The listing builds one solid part. Answer for the finished solid, in the listing's coordinates (mm). Face numbers are marked on the shaded views. A direction names the side the tool comes from. Give positions to 0.01 mm unless a question says otherwise; leave off trailing zeros. Write each loop counter-clockwise with the first axis right and the second up, starting at its lowest first coordinate (ties: lowest second). Pieces come first, ordered by that corner, then holes. Notation, with made-up numbers: M -25,-17 L 26,-17 A16 ccw 26,-1 Z; hole C 78,79 d2. An arc over 180 degrees is marked long. Return JSON: item names as keys, results as strings.
from build123d import *

# Parameters (mm, degrees)
F1_DEPTH     = 25.4
F2_R         = 9.525
F3_DEPTH     = 42.7816898715
F4_R         = 25.39999
F5_R         = 3.175
F6_W         = 5.0767767243
F6_H         = 5.0767767243
F7_DEPTH     = 3.175
F8_T1_DEPTH  = 142.613798458
F8_T3_DEPTH  = 25.40001
F8_T5_DEPTH  = 44.45
F8_T7_DEPTH  = 25.40001
F8_T9_DEPTH  = 2e-05
F8_T12_ANGLE = 90
F8_T14_ANGLE = 55
F8_T16_ANGLE = 55
F8_T18_ANGLE = 90
F8_T20_ANGLE = 90
F8_T22_ANGLE = 90
F8_T24_ANGLE = 55
F8_T26_ANGLE = 90
F8_T28_ANGLE = 90
F8_T30_ANGLE = 90
F8_T32_ANGLE = 55
F8_T34_ANGLE = 90


# Not quite as in the source:
# - a fillet or chamfer that OpenCascade refuses, or shapes differently, is made with other operations: its cross-section is extruded or revolved along the edge and cut away or added
# - a fillet or chamfer is up to 0.001 mm smaller than in the source, because OpenCascade refuses the exact size


with BuildPart() as f1:
    # F0 (on Front) → F1 (new body, symmetric)
    with BuildSketch(Plane.XZ):
        with BuildLine():
            Line((118.9895820573, 10.6313137069), (-26.7992164007, 10.6313137069))
            Line((-26.7992164007, 10.6313137069), (-26.7992164007, -2.0686862931))
            Line((-26.7992164007, -2.0686862931), (118.9895820573, -2.0686862931))
            ThreePointArc((118.9895820573, -2.0686862931), (130.7179968335, 0.8012385441), (139.7960439822, 8.7624722235))
            Line((139.7960439822, 8.7624722235), (168.9337269489, 50.3753960734))
            Line((168.9337269489, 50.3753960734), (158.5304959864, 57.6598168151))
            Line((158.5304959864, 57.6598168151), (129.3928130198, 16.0468929652))
            ThreePointArc((129.3928130198, 16.0468929652), (124.8537894454, 12.0662761255), (118.9895820573, 10.6313137069))
        make_face()
    extrude(amount=F1_DEPTH, both=True)

    # F2 (on face) → F3 (cut, through all)
    with BuildSketch(Plane(origin=(79.2843072841, 0, -55.515469622), x_dir=(0, -1, 0), z_dir=(-0.8191520443, 0, 0.5735764364))):
        with Locations((0, 115.9365137582)):
            Circle(F2_R)
    extrude(amount=-F3_DEPTH, mode=Mode.SUBTRACT)

    # F4 (radius 25.4 in the source; OpenCascade refuses exactly that, so slightly less here)
    f4_edges = [f1.edges().sort_by_distance(p)[0] for p in [
        (163.732111, 25.4, 54.017606),
        (163.732111, -25.4, 54.017606),
    ]]
    fillet(f4_edges, radius=F4_R)

    # F5
    f5_edges = [f1.edges().sort_by_distance(p)[0] for p in [
        (-26.799216, -25.4, 4.281314),
        (-26.799216, 25.4, 4.281314),
    ]]
    fillet(f5_edges, radius=F5_R)

    # F6 (on face) → F7 (cut)
    with BuildSketch(Plane(origin=(0, 0, -2.0686862931), x_dir=(1, 0, 0), z_dir=(0, 0, -1))):
        with Locations((4.9507835993, 0)):
            Rectangle(F6_W, F6_H)
    extrude(amount=-F7_DEPTH, mode=Mode.SUBTRACT)

    # F8: fillet of radius 3.175 on 24 edges, made by hand

    # F8_s2 → F8_t1 (cut)
    with BuildSketch(Plane.YZ.offset(-23.6242164007)):
        with BuildLine():
            ThreePointArc((25.4, 7.4563137069), (24.4700640303, 9.7013777371), (22.225, 10.6313137069))
            Line((22.225, 10.6313137069), (25.4, 10.6313137069))
            Line((25.4, 10.6313137069), (25.4, 7.4563137069))
        make_face()
        with BuildLine():
            ThreePointArc((-22.225, 10.6313137069), (-24.4700640303, 9.7013777371), (-25.4, 7.4563137069))
            Line((-25.4, 7.4563137069), (-25.4, 10.6313137069))
            Line((-25.4, 10.6313137069), (-22.225, 10.6313137069))
        make_face()
        with BuildLine():
            ThreePointArc((-22.225, -2.0686862931), (-24.4700640303, -1.1387503234), (-25.4, 1.1063137069))
            Line((-25.4, 1.1063137069), (-25.4, -2.0686862931))
            Line((-25.4, -2.0686862931), (-22.225, -2.0686862931))
        make_face()
        with BuildLine():
            ThreePointArc((25.4, 1.1063137069), (24.4700640303, -1.1387503234), (22.225, -2.0686862931))
            Line((22.225, -2.0686862931), (25.4, -2.0686862931))
            Line((25.4, -2.0686862931), (25.4, 1.1063137069))
        make_face()
    extrude(amount=F8_T1_DEPTH, mode=Mode.SUBTRACT)

    # F8_s4 → F8_t3 (cut)
    with BuildSketch(Plane(origin=(64.6773529548, 0, 92.3688327037), x_dir=(0, 1, 0), z_dir=(-0.5735764364, 0, -0.8191520443))):
        with BuildLine():
            ThreePointArc((25.4, 99.96326762), (24.4700640303, 97.7182035897), (22.225, 96.78826762))
            Line((22.225, 96.78826762), (25.4, 96.78826762))
            Line((25.4, 96.78826762), (25.4, 99.96326762))
        make_face()
        with BuildLine():
            ThreePointArc((-22.225, 96.78826762), (-24.4700640303, 97.7182035897), (-25.4, 99.96326762))
            Line((-25.4, 99.96326762), (-25.4, 96.78826762))
            Line((-25.4, 96.78826762), (-22.225, 96.78826762))
        make_face()
    extrude(amount=F8_T3_DEPTH, mode=Mode.SUBTRACT)

    # F8_s6 → F8_t5 (cut)
    with BuildSketch(Plane.XZ.offset(-22.225)):
        with BuildLine():
            ThreePointArc((-23.6242164007, 10.6313137069), (-25.869280431, 9.7013777371), (-26.7992164007, 7.4563137069))
            Line((-26.7992164007, 7.4563137069), (-26.7992164007, 10.6313137069))
            Line((-26.7992164007, 10.6313137069), (-23.6242164007, 10.6313137069))
        make_face()
        with BuildLine():
            ThreePointArc((-23.6242164007, -2.0686862931), (-25.869280431, -1.1387503234), (-26.7992164007, 1.1063137069))
            Line((-26.7992164007, 1.1063137069), (-26.7992164007, -2.0686862931))
            Line((-26.7992164007, -2.0686862931), (-23.6242164007, -2.0686862931))
        make_face()
    extrude(amount=F8_T5_DEPTH, mode=Mode.SUBTRACT)

    # F8_s8 → F8_t7 (cut)
    with BuildSketch(Plane(origin=(50.1085057357, 0, 71.5623625873), x_dir=(0, 1, 0), z_dir=(0.5735764364, 0, 0.8191520443))):
        with BuildLine():
            ThreePointArc((25.4, -106.31326762), (24.4700640303, -108.5583316502), (22.225, -109.48826762))
            Line((22.225, -109.48826762), (25.4, -109.48826762))
            Line((25.4, -109.48826762), (25.4, -106.31326762))
        make_face()
        with BuildLine():
            ThreePointArc((-22.225, -109.48826762), (-24.4700640303, -108.5583316502), (-25.4, -106.31326762))
            Line((-25.4, -106.31326762), (-25.4, -109.48826762))
            Line((-25.4, -109.48826762), (-22.225, -109.48826762))
        make_face()
    extrude(amount=F8_T7_DEPTH, mode=Mode.SUBTRACT)

    # F8_s10 → F8_t9 (cut)
    with BuildSketch(Plane.XZ.offset(-1e-05)):
        with BuildLine():
            ThreePointArc((167.1126217635, 47.7745883328), (167.6385786386, 50.1470264823), (166.3329192083, 52.1965012588))
            Line((166.3329192083, 52.1965012588), (168.9337269489, 50.3753960734))
            Line((168.9337269489, 50.3753960734), (167.1126217635, 47.7745883328))
        make_face()
        with BuildLine():
            ThreePointArc((156.709390801, 55.0590090745), (158.7588655775, 56.3646685049), (161.131303727, 55.8387116297))
            Line((161.131303727, 55.8387116297), (158.5304959864, 57.6598168151))
            Line((158.5304959864, 57.6598168151), (156.709390801, 55.0590090745))
        make_face()
    extrude(amount=F8_T9_DEPTH, mode=Mode.SUBTRACT)

    # F8_s11 → F8_t12 (revolve, cut)
    with BuildSketch(Plane(origin=(64.6773529548, 0, 92.3688327037), x_dir=(0, 1, 0), z_dir=(-0.5735764364, 0, -0.8191520443))):
        with BuildLine():
            ThreePointArc((25.4, 99.96326762), (24.4700640303, 97.7182035897), (22.225, 96.78826762))
            Line((22.225, 96.78826762), (25.4, 96.78826762))
            Line((25.4, 96.78826762), (25.4, 99.96326762))
        make_face()
    revolve(axis=Axis((143.9616602388, 1e-05, 36.8533630817), (0.8191520443, 0, -0.5735764364)), revolution_arc=F8_T12_ANGLE, mode=Mode.SUBTRACT)

    # F8_s13 → F8_t14 (revolve, cut)
    with BuildSketch(Plane.YZ.offset(118.9895820573)):
        with BuildLine():
            ThreePointArc((25.4, 1.1063137069), (24.4700640303, -1.1387503234), (22.225, -2.0686862931))
            Line((22.225, -2.0686862931), (25.4, -2.0686862931))
            Line((25.4, -2.0686862931), (25.4, 1.1063137069))
        make_face()
    revolve(axis=Axis((118.9895820573, 25.4, 23.3313137069), (0, -1, 0)), revolution_arc=F8_T14_ANGLE, mode=Mode.SUBTRACT)

    # F8_s15 → F8_t16 (revolve, cut)
    with BuildSketch(Plane(origin=(50.1085057357, 0, 71.5623625873), x_dir=(0, 1, 0), z_dir=(0.5735764364, 0, 0.8191520443))):
        with BuildLine():
            ThreePointArc((25.4, -99.96326762), (24.4700640303, -97.7182035897), (22.225, -96.78826762))
            Line((22.225, -96.78826762), (25.4, -96.78826762))
            Line((25.4, -96.78826762), (25.4, -99.96326762))
        make_face()
    revolve(axis=Axis((118.9895820573, 25.4, 23.3313137069), (0, 1, 0)), revolution_arc=F8_T16_ANGLE, mode=Mode.SUBTRACT)

    # F8_s17 → F8_t18 (revolve, cut)
    with BuildSketch(Plane.YZ.offset(-23.6242164007)):
        with BuildLine():
            ThreePointArc((22.225, -2.0686862931), (24.4700640303, -1.1387503234), (25.4, 1.1063137069))
            Line((25.4, 1.1063137069), (25.4, -2.0686862931))
            Line((25.4, -2.0686862931), (22.225, -2.0686862931))
        make_face()
    revolve(axis=Axis((-23.6242164007, 22.225, -2.0686862931), (0, 0, 1)), revolution_arc=F8_T18_ANGLE, mode=Mode.SUBTRACT)

    # F8_s19 → F8_t20 (revolve, cut)
    with BuildSketch(Plane.YZ.offset(-23.6242164007)):
        with BuildLine():
            ThreePointArc((-22.225, -2.0686862931), (-24.4700640303, -1.1387503234), (-25.4, 1.1063137069))
            Line((-25.4, 1.1063137069), (-25.4, -2.0686862931))
            Line((-25.4, -2.0686862931), (-22.225, -2.0686862931))
        make_face()
    revolve(axis=Axis((-23.6242164007, -22.225, -2.0686862931), (0, 0, -1)), revolution_arc=F8_T20_ANGLE, mode=Mode.SUBTRACT)

    # F8_s21 → F8_t22 (revolve, cut)
    with BuildSketch(Plane.YZ.offset(-23.6242164007)):
        with BuildLine():
            ThreePointArc((25.4, 7.4563137069), (24.4700640303, 9.7013777371), (22.225, 10.6313137069))
            Line((22.225, 10.6313137069), (25.4, 10.6313137069))
            Line((25.4, 10.6313137069), (25.4, 7.4563137069))
        make_face()
    revolve(axis=Axis((-23.6242164007, 22.225, 10.6313137069), (0, 0, 1)), revolution_arc=F8_T22_ANGLE, mode=Mode.SUBTRACT)

    # F8_s23 → F8_t24 (revolve, cut)
    with BuildSketch(Plane.YZ.offset(118.9895820573)):
        with BuildLine():
            ThreePointArc((-22.225, -2.0686862931), (-24.4700640303, -1.1387503234), (-25.4, 1.1063137069))
            Line((-25.4, 1.1063137069), (-25.4, -2.0686862931))
            Line((-25.4, -2.0686862931), (-22.225, -2.0686862931))
        make_face()
    revolve(axis=Axis((118.9895820573, -25.4, 23.3313137069), (0, -1, 0)), revolution_arc=F8_T24_ANGLE, mode=Mode.SUBTRACT)

    # F8_s25 → F8_t26 (revolve, cut)
    with BuildSketch(Plane.YZ.offset(-23.6242164007)):
        with BuildLine():
            ThreePointArc((-22.225, 10.6313137069), (-24.4700640303, 9.7013777371), (-25.4, 7.4563137069))
            Line((-25.4, 7.4563137069), (-25.4, 10.6313137069))
            Line((-25.4, 10.6313137069), (-22.225, 10.6313137069))
        make_face()
    revolve(axis=Axis((-23.6242164007, -22.225, 10.6313137069), (0, 0, -1)), revolution_arc=F8_T26_ANGLE, mode=Mode.SUBTRACT)

    # F8_s27 → F8_t28 (revolve, cut)
    with BuildSketch(Plane(origin=(64.6773529548, 0, 92.3688327037), x_dir=(0, 1, 0), z_dir=(-0.5735764364, 0, -0.8191520443))):
        with BuildLine():
            ThreePointArc((22.225, 109.48826762), (24.4700640303, 108.5583316502), (25.4, 106.31326762))
            Line((25.4, 106.31326762), (25.4, 109.48826762))
            Line((25.4, 109.48826762), (22.225, 109.48826762))
        make_face()
    revolve(axis=Axis((154.3648912013, 1e-05, 29.56894234), (0.8191520443, 0, -0.5735764364)), revolution_arc=F8_T28_ANGLE, mode=Mode.SUBTRACT)

    # F8_s29 → F8_t30 (revolve, cut)
    with BuildSketch(Plane.XZ.offset(1e-05)):
        with BuildLine():
            ThreePointArc((167.1126217635, 47.7745883328), (167.6385786386, 50.1470264823), (166.3329192083, 52.1965012588))
            Line((166.3329192083, 52.1965012588), (168.9337269489, 50.3753960734))
            Line((168.9337269489, 50.3753960734), (167.1126217635, 47.7745883328))
        make_face()
    revolve(axis=Axis((154.3648912013, -1e-05, 29.56894234), (0.8191520443, 0, -0.5735764364)), revolution_arc=F8_T30_ANGLE, mode=Mode.SUBTRACT)

    # F8_s31 → F8_t32 (revolve, cut)
    with BuildSketch(Plane(origin=(50.1085057357, 0, 71.5623625873), x_dir=(0, 1, 0), z_dir=(0.5735764364, 0, 0.8191520443))):
        with BuildLine():
            ThreePointArc((-22.225, -96.78826762), (-24.4700640303, -97.7182035897), (-25.4, -99.96326762))
            Line((-25.4, -99.96326762), (-25.4, -96.78826762))
            Line((-25.4, -96.78826762), (-22.225, -96.78826762))
        make_face()
    revolve(axis=Axis((118.9895820573, -25.4, 23.3313137069), (0, 1, 0)), revolution_arc=F8_T32_ANGLE, mode=Mode.SUBTRACT)

    # F8_s33 → F8_t34 (revolve, cut)
    with BuildSketch(Plane.XZ.offset(1e-05)):
        with BuildLine():
            ThreePointArc((156.709390801, 55.0590090745), (158.7588655775, 56.3646685049), (161.131303727, 55.8387116297))
            Line((161.131303727, 55.8387116297), (158.5304959864, 57.6598168151))
            Line((158.5304959864, 57.6598168151), (156.709390801, 55.0590090745))
        make_face()
    revolve(axis=Axis((143.9616602388, -1e-05, 36.8533630817), (0.8191520443, 0, -0.5735764364)), revolution_arc=F8_T34_ANGLE, mode=Mode.SUBTRACT)


solid = f1.part
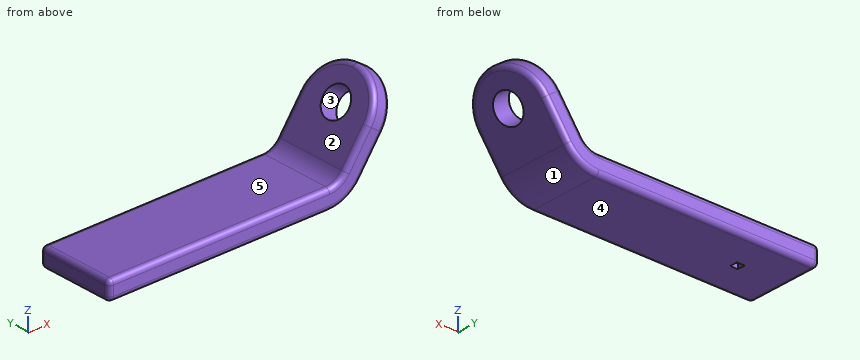
Item 1: Which of the six approach directions +Z, -Z, +X, -X, +Y, -Y give full straight-line access (tool end or side, diameter ignored) to the marked faces 4 and 5?
Geometry results:
{"face 4": "-Z, +X, -X, +Y, -Y", "face 5": "+Z, -X, +Y, -Y"}
Item 2: Given pin 1 Ø5.5 at (x, y) = (5.5, 0) entering from -Z; pin 2 Ø4 at (y, z) = (-14, 25) entering from +X; pin 3 Ø3.5 at (y, z) = (-1, -0.5) entering from +X; pin 4 Ø3 at (y, z) = (6.5, 24) entering from +X, each flat-ended and moving along its own axis, determine where each tip first touches the part or whether it passes through.
Geometry results:
{"pin 1": "stops at z = -2.07", "pin 2": "stops at x = 152.57", "pin 3": "stops at x = 131.54", "pin 4": "stops at x = 151.52"}
Item 3: Find the intervals of material crossed by line 1 (Z direction, x = 3, y = 18); line 2 (Z direction, x = 130.5, y = -1); line 3 (X direction, y = 19.5, z = 37), in increasing order.
Geometry results:
{"line 1": "z = -2.07 to 10.63", "line 2": "z = 0.69 to 17.63", "line 3": "x = 144.06 to 159.57"}
Item 4: Determine the mould class of the marked faces 1, 2 and 3 for opening direction Z: +Z half, -Z half, draft (parallel to the pull), parting line (faces both ways), or undercut.
Geometry results:
{"face 1": "-Z half", "face 2": "+Z half", "face 3": "undercut"}
Item 5: A cutting plane is placed at A-A, the plane x = 10.5. Write down the section's boundary in (y, z) (3 decimals).
Geometry results:
{"outline": "M -25.4,1.106 A3.175 ccw -22.225,-2.069 L 22.225,-2.069 A3.175 ccw 25.4,1.106 L 25.4,7.456 A3.175 ccw 22.225,10.631 L -22.225,10.631 A3.175 ccw -25.4,7.456 Z"}
